Geometry check sheet. Reference: drawing and pictorial views, mm from the part's lowest x, y, z. Round coordinates to 2 decimals unless told otherwise and drop trailing zeros. Order: outer loops, then holes, each group sorted by start corner. A loop starts at its lowest first (then second) coordinate and runs counter-clockwise, first axis right, second up.
(1) Cross-section at B-B on x = 202.5. Enter the section's corners in (y, z).
(2) Cross-section at A-A on y = 1.1. Enter the section's corners in (x, z).
(3) Cross-section at C-C on x = 367.5. Enter the section's corners in (y, z).
(4) Cross-section at D-D on z = 163. Enter the section's corners in (x, y), and give its area (3 significant figures).
(5) Thickness scan on L1, parallel to X at y = 2.1, z = 289; L2, parallel to Z at x = 321, y = 2.3; L3, parallel to Z at x = 341, y = 3.85. Record the ranges inside material, lowest first.
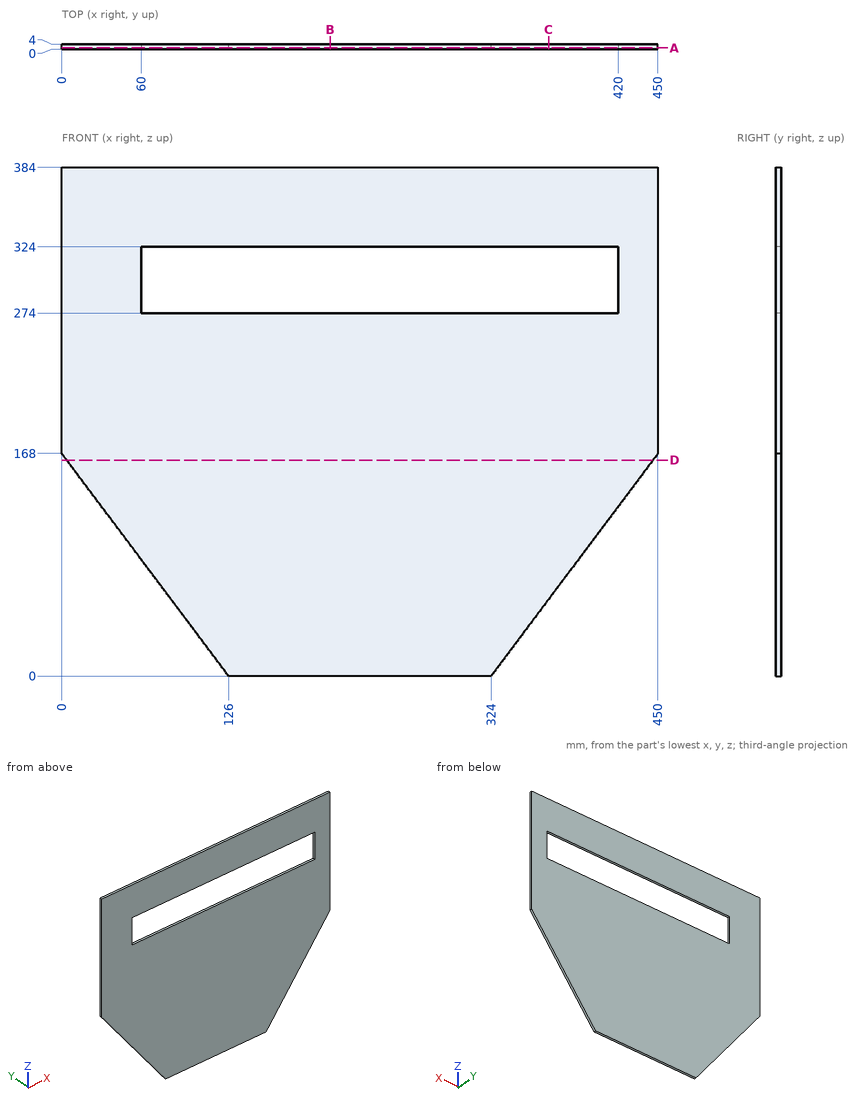
Found:
1. outline: (0, 0) - (4, 0) - (4, 274) - (0, 274) - close; (0, 324) - (4, 324) - (4, 384) - (0, 384) - close
2. outline: (0, 168) - (126, 0) - (324, 0) - (450, 168) - (450, 384) - (0, 384) - close; hole (60, 274) - (420, 274) - (420, 324) - (60, 324) - close
3. outline: (0, 58) - (4, 58) - (4, 274) - (0, 274) - close; (0, 324) - (4, 324) - (4, 384) - (0, 384) - close
4. outline: (3.75, 0) - (446.25, 0) - (446.25, 4) - (3.75, 4) - close
4. area: 1,770 mm2
5. L1: x = 0 to 60, 420 to 450
5. L2: z = 0 to 274, 324 to 384
5. L3: z = 22.67 to 274, 324 to 384
